```python
from build123d import *

# Parameters (mm, degrees)
F0_R     = 10.5
F0_R_2   = 5.5
F2_DEPTH = 2.5
F1_R     = 5.5
F1_R_2   = 4.075
F3_DEPTH = 3
F4_DEPTH = 5.5
F5_R     = 0.8


with BuildPart() as f2:
    # F0 (on Front) → F2 (new body)
    with BuildSketch(Plane.XZ):
        Circle(F0_R)
        Circle(F0_R_2, mode=Mode.SUBTRACT)
    extrude(amount=F2_DEPTH)

    # F1 (on face) → F3 (join)
    with BuildSketch(Plane.XZ):
        Circle(F1_R)
        Circle(F1_R_2, mode=Mode.SUBTRACT)
    extrude(amount=F3_DEPTH)

    # F1 (on face) → F4 (join)
    with BuildSketch(Plane.XZ):
        Circle(F1_R_2)
    extrude(amount=F4_DEPTH)

    # F5
    f5_edges = [f2.edges().sort_by_distance(p)[0] for p in [
        (-10.5, 0, 0),
        (-10.5, -2.5, 0),
    ]]
    fillet(f5_edges, radius=F5_R)


solid = f2.part
```
CAD build for the part. Positions are in the model's coordinates, mm. A direction names the side the tool comes from. Round coordinates to 2 decimals unless told otherwise and drop trailing zeros. Order: outer loops, then holes, each group sorted by start corner. A loop starts at its lowest first (then second) coordinate and runs counter-clockwise, first axis right, second up.
Q1. Drop flat-ended pins along their axis: pin 1 (1 mm diameter, centred on x = 2.5, y = -1.5, fed in from +Z); pin 2 (2 mm diameter, centred on x = 6.5, y = -2, fed in from +Z); pin 3 (3 mm diameter, centred on x = 0, z = -7, fed in from +Y). Give the stop position or say it passes through.
Q2. Slice it at C-C (y = -4.3). Write the cut outline in (x, z) (3 decimals).
Q3. Slice it at A-A (z = 0). Write the cut outline in (x, y) (3 decimals), and give its area (3 significant figures).
Q4. Which spindle directions (+Z, -Z, +X, -X, +Y, -Y) get a long thin tool onto all of the face, cutting with end or side? Do faces 1 (the cylindrical face through (10, -1.2, 3.2)), 2 (the cylindrical face through (-1.19, -2.75, -5.37)). Say none if no direction does.
Q5. Wall check: L1, parallel to Y at x = -8, z = -3; L2, parallel to Z at x = 3.5, y = -0.8; L3, parallel to Z at x = 3.75, y = -4.5. Give the ranges that are in metal, low to high.
Q6. Slice it at B-B (x = 0). Write the cut outline in (y, z) (3 decimals), and give its area (3 significant figures).
Results below:
1. pin 1: stops at z = 10.31
1. pin 2: stops at z = 8.92
1. pin 3: stops at y = 0
2. outline: circle Ø8.15 at (0, 0)
3. outline: (-10.5, -1.7) arc R0.8 ccw to (-9.7, -2.5) - (-5.5, -2.5) - (-5.5, -3) - (-4.075, -3) - (-4.075, -5.5) - (4.075, -5.5) - (4.075, -3) - (5.5, -3) - (5.5, -2.5) - (9.7, -2.5) arc R0.8 ccw to (10.5, -1.7) - (10.5, -0.8) arc R0.8 ccw to (9.7, 0) - (-9.7, 0) arc R0.8 ccw to (-10.5, -0.8) - close
3. area: 77.8 mm2
4. face 1: +Y, -Y
4. face 2: -Y
5. L1: y = -2.5 to 0
5. L2: z = -9.9 to 9.9
5. L3: z = -1.59 to 1.59
6. outline: (-5.5, -4.075) - (-3, -4.075) - (-3, -5.5) - (-2.5, -5.5) - (-2.5, -9.7) arc R0.8 ccw to (-1.7, -10.5) - (-0.8, -10.5) arc R0.8 ccw to (0, -9.7) - (0, 9.7) arc R0.8 ccw to (-0.8, 10.5) - (-1.7, 10.5) arc R0.8 ccw to (-2.5, 9.7) - (-2.5, 5.5) - (-3, 5.5) - (-3, 4.075) - (-5.5, 4.075) - close
6. area: 77.8 mm2
